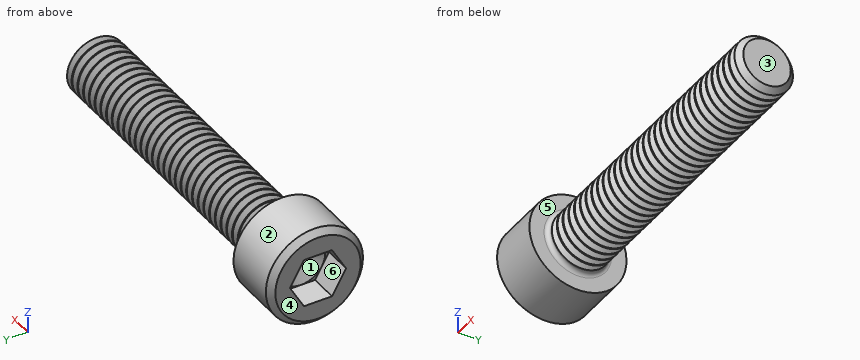
```python
from build123d import *

# Parameters (mm, degrees)
FILLET1_R       = 0.3556
HEX_2_DEPTH     = 2.286
THDSCHPAT_COUNT = 32
THDSCHPAT_PITCH = 0.768985


with BuildPart() as part:
    # BodySke → Base-Revolve (revolve)
    with BuildSketch(Plane.XY, mode=Mode.PRIVATE) as base_revolve_sk:
        Polygon((0, 0), (0, 3.48615), (0.4826, 3.96875), (4.826, 3.96875), (4.826, 2.413), (29.75356, 2.413), (30.226, 1.94056), (30.226, 0), align=None)
    revolve(base_revolve_sk.sketch.rotate(Axis((-31.75, 0, 0), (1, 0, 0)), 90), axis=Axis((-31.75, 0, 0), (1, 0, 0)))

    # Fillet1
    fillet1_edges = [part.edges().sort_by_distance(p)[0] for p in [
        (4.826, 0, -2.413),
    ]]
    fillet(fillet1_edges, radius=FILLET1_R)

    # Sketch2 → Hex-PreBroach (revolve, cut)
    with BuildSketch(Plane.XY, mode=Mode.PRIVATE) as hex_prebroach_sk:
        Polygon((0, 1.98501), (2.286, 1.98501), (3.432046058, 0), (0, 0), align=None)
    revolve(hex_prebroach_sk.sketch.rotate(Axis((0, 0, 0), (1, 0, 0)), 90), axis=Axis((0, 0, 0), (1, 0, 0)), mode=Mode.SUBTRACT)

    # Sketch3 → Hex 2 (cut)
    with BuildSketch(Plane(origin=(0, 0, 0), x_dir=(0, 0.500000000000001, 0.866025403784438), z_dir=(-1, 0, 0))):
        Polygon((1.146046058, 1.98501), (-1.146046058, 1.98501), (-2.292092116, 0), (-1.146046058, -1.98501), (1.146046058, -1.98501), (2.292092116, 0), align=None)
    extrude(amount=-HEX_2_DEPTH, mode=Mode.SUBTRACT)

    # ThdSchSke → ThreadSchematic (revolve, cut)
    with BuildSketch(Plane.XY):
        Polygon((5.61848, -1.94056), (5.287673951, -2.413), (5.287673951, -3.01625), (5.949286049, -3.01625), (5.949286049, -2.413), align=None)
    threadschematic = revolve(axis=Axis((-3.175, 0, 0), (1, 0, 0)), mode=Mode.SUBTRACT)

    # ThdSchPat: ThreadSchematic ×32
    with Locations(*[(i * THDSCHPAT_PITCH, 0, 0) for i in range(1, THDSCHPAT_COUNT)]):
        add(threadschematic, mode=Mode.SUBTRACT)


solid = part.part
```
Geometry: final body of the model. Coordinates: model frame, mm. Face numbers are marked on the shaded views. A direction names the side the tool comes from. Round coordinates to 2 decimals unless told otherwise and drop trailing zeros. Write each question's results on one line, items separated by ' | '.
Q1. Ray query, line 1 along X through (y, z) = (-0.75, 3); line 2 along X through (y, z) = (-0.75, 0.25); line 3 along Z through (x, y) = (18.5, -1.75). Return the intervals inside material, ascending.
Response values:
line 1: 0 to 4.83 | line 2: 2.98 to 30.23 | line 3: -1.36 to 1.36
Q2. Access query for the marked faces 4, 5 and 6. Directions: +Z, -Z, +X, -X, +Y, -Y. A direction counts if a zero-diameter tool reaches every point of the face in a straight line with its end or side. Return the directions, or none.
Response values:
face 4: +Z, -Z, -X, +Y, -Y | face 5: +X | face 6: -X
Q3. Pin query (flat end, axial travel): pin 1 Ø3 at (x, z) = (12.5, -2.5) entering from +Y; pin 2 Ø0.5 at (y, z) = (-1, -1.5) entering from -X; pin 3 Ø1.5 at (y, z) = (-1, 2) entering from -X; pin 4 Ø3 at (x, y) = (8, 1.5) entering from -Z. Return the tip coordinate at first contact, or that it passes through.
Response values:
pin 1: y = 2.18 | pin 2: x = 2.29 | pin 3: x = 0 | pin 4: z = -2.41
Q4. Pull-direction query (Y, two-part tool) for the marked faces 1, 2 and 3; classes: released by +Y, released by -Y, zero draft, split by the parting line, or undercut.
Response values:
face 1: undercut | face 2: split by the parting line | face 3: zero draft
